For this review, take the finished solid that the model builds, in its own axes (mm). Face numbers are marked on the shaded views. A direction names the side the tool comes from. Coordinates: 2 decimals unless noted, no trailing zeros. Loops run counter-clockwise (first coordinate to the right, second up) from the corner with the lowest first, then second, coordinate; pieces in that order, holes last. Notation, with made-up numbers: (-39, 46) -> (-25, 46) arc R15 ccw to (-25, 51) -> close; hole circle Ø5 at (-12, 73). An arc over 180 degrees is marked (long way). Answer in a Markdown table with one row per item.
from build123d import *

# Parameters (mm, degrees)
F0_R     = 1.5
F1_DEPTH = 5
F2_R     = 1.5
F3_DEPTH = 40.501
F4_SIZE  = 1
F5_R     = 5
F7_W     = 44.468724
F7_H     = 10
F8_DEPTH = 3


with BuildPart() as f1:
    # F0 (on Top) → F1 (new body, symmetric)
    with BuildSketch(Plane.XY):
        with BuildLine():
            ThreePointArc((2.5, 17.825543), (17.956333, -1.25304), (0, -18))
            ThreePointArc((0, -18), (-17.956333, -1.25304), (-2.5, 17.825543))
            Line((-2.5, 17.825543), (-2.5, 27.825543))
            Line((-2.5, 27.825543), (-12.5, 27.825543))
            Line((-12.5, 27.825543), (-12.5, 20.825543))
            Line((-12.5, 20.825543), (-18.716216, 20.825543))
            ThreePointArc((-18.716216, 20.825543), (-27.902736, -2.331809), (-15, -23.643181))
            Line((-15, -23.643181), (-15, -54.25))
            Line((-15, -54.25), (0, -54.25))
            Line((0, -54.25), (15, -54.25))
            Line((15, -54.25), (15, -23.643181))
            ThreePointArc((15, -23.643181), (27.902736, -2.331809), (18.716216, 20.825543))
            Line((18.716216, 20.825543), (12.5, 20.825543))
            Line((12.5, 20.825543), (12.5, 27.825543))
            Line((12.5, 27.825543), (2.5, 27.825543))
            Line((2.5, 27.825543), (2.5, 17.825543))
        make_face()
        with Locations((-11, -40)):
            Circle(F0_R, mode=Mode.SUBTRACT)
        with Locations((0, -51)):
            Circle(F0_R, mode=Mode.SUBTRACT)
        with Locations((11, -40)):
            Circle(F0_R, mode=Mode.SUBTRACT)
        with Locations((0, -29)):
            Circle(F0_R, mode=Mode.SUBTRACT)
    extrude(amount=F1_DEPTH, both=True)

    # F2 (on face) → F3 (cut, through all)
    with BuildSketch(Plane(origin=(-12.5, 0, 0), x_dir=(0, -1, 0), z_dir=(-1, 0, 0))):
        with Locations((-24.325543, 0)):
            Circle(F2_R)
    extrude(amount=-F3_DEPTH, mode=Mode.SUBTRACT)

    # F4
    f4_edges = [f1.edges().sort_by_distance(p)[0] for p in [
        (12.5, 27.825543, 0),
        (-12.5, 27.825543, 0),
    ]]
    chamfer(f4_edges, length=F4_SIZE)

    # F5
    f5_edges = [f1.edges().sort_by_distance(p)[0] for p in [
        (-15, -54.25, 0),
        (15, -54.25, 0),
    ]]
    fillet(f5_edges, radius=F5_R)

    # F7 (on plane+point) → F8 (cut)
    with BuildSketch(Plane.YZ.offset(-28)):
        with Locations((-1.408819, 0)):
            Rectangle(F7_W, F7_H)
    extrude(amount=F8_DEPTH, mode=Mode.SUBTRACT)


solid = f1.part
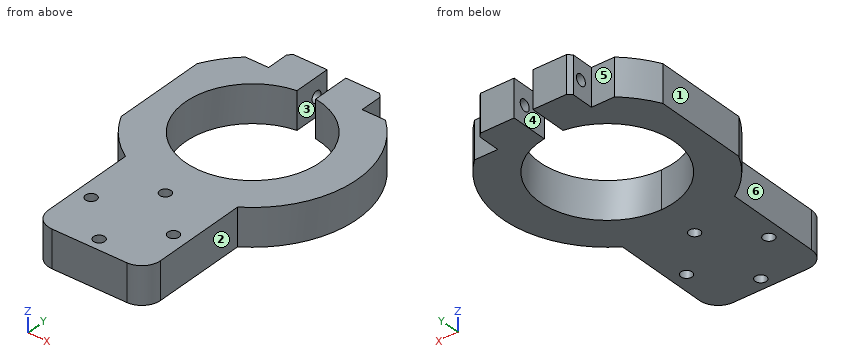
Item 1: Take a section at A-A, the plane z = 0. Count the separate pieces of the cut face and the enclosed holes in it, and give its area (3 significant figures).
Worked answers:
| item | result |
|---|---|
| separate pieces | 3 |
| enclosed holes | 4 |
| area | 2,070 mm² |
Item 2: The part is to be moulded in two halves that separate along X. For the marked faces 4, 5 and 6, say which applies: +X half, -X half, draft (parallel to the pull), parting line (faces both ways), or undercut.
Worked answers:
| item | result |
|---|---|
| face 4 | undercut |
| face 5 | draft |
| face 6 | -X half |
Item 3: Take a section at C-C, the plane y = -29. State the section outline as (x, z) points.
Worked answers:
| item | result |
|---|---|
| outline | (-15, -5) -> (-1.5, -5) -> (-1.5, 5) -> (-15, 5) -> close; (1.5, -5) -> (15, -5) -> (15, 5) -> (1.5, 5) -> close |
Item 4: For the marked faces 1, 2 and 3, list the 3-axis set-ups (+Z, -Z, +X, -X, +Y, -Y) from which the entire face can be reached by the end or side of a thin tool; tool diameter is ignored.
Worked answers:
| item | result |
|---|---|
| face 1 | +Z, -Z, -X, +Y, -Y |
| face 2 | +Z, -Z, +X, -Y |
| face 3 | +Z, -Z, +Y |
Item 5: Take a section at B-B, the plane y = -40. State the section outline as (x, z) points.
Worked answers:
| item | result |
|---|---|
| outline | (-15, -5) -> (-12.5, -5) -> (-12.5, 5) -> (-15, 5) -> close; (-9.5, -5) -> (9.5, -5) -> (9.5, 5) -> (-9.5, 5) -> close; (12.5, -5) -> (15, -5) -> (15, 5) -> (12.5, 5) -> close |
Item 6: For L1, parallel to X at y = 24.5, z = -3.5; L2, parallel to X at y = -5, z = -2.5; L3, parallel to Y at x = 16, z = -1.75, list the stretches that pass through material, from the lowest coordinate up.
Worked answers:
| item | result |
|---|---|
| L1 | -12.5 to -2.5, 2.5 to 12.5 |
| L2 | -25 to -17.29, 17.29 to 27.55 |
| L3 | -22.98 to -8.25, 8.25 to 20.83 |
Item 7: Insertion check: pin 1 (3 mm diameter, centred on x = -16, z = -1.5, fed in from +Y); pin 2 (5 mm diameter, centred on y = -10.5, z = -1, fed in from +X); pin 3 (5 mm diameter, centred on y = 23.5, z = -0.5, fed in from +X). Each pin has a flat end and moves straight along its axis. Give the tip position at first contact, or say it passes through.
Worked answers:
| item | result |
|---|---|
| pin 1 | y = 20.83 |
| pin 2 | x = 26.83 |
| pin 3 | x = 12.5 |
Item 8: Take a section at D-D, the plane x = -5. State the section outline as (y, z) points, and give its area (3 significant figures).
Worked answers:
| item | result |
|---|---|
| outline | (-54.25, -5) -> (-17.29, -5) -> (-17.29, 5) -> (-54.25, 5) -> close; (17.29, -5) -> (27.83, -5) -> (27.83, 5) -> (17.29, 5) -> close; hole circle Ø3 at (24.33, 0) |
| area | 468 mm² |
